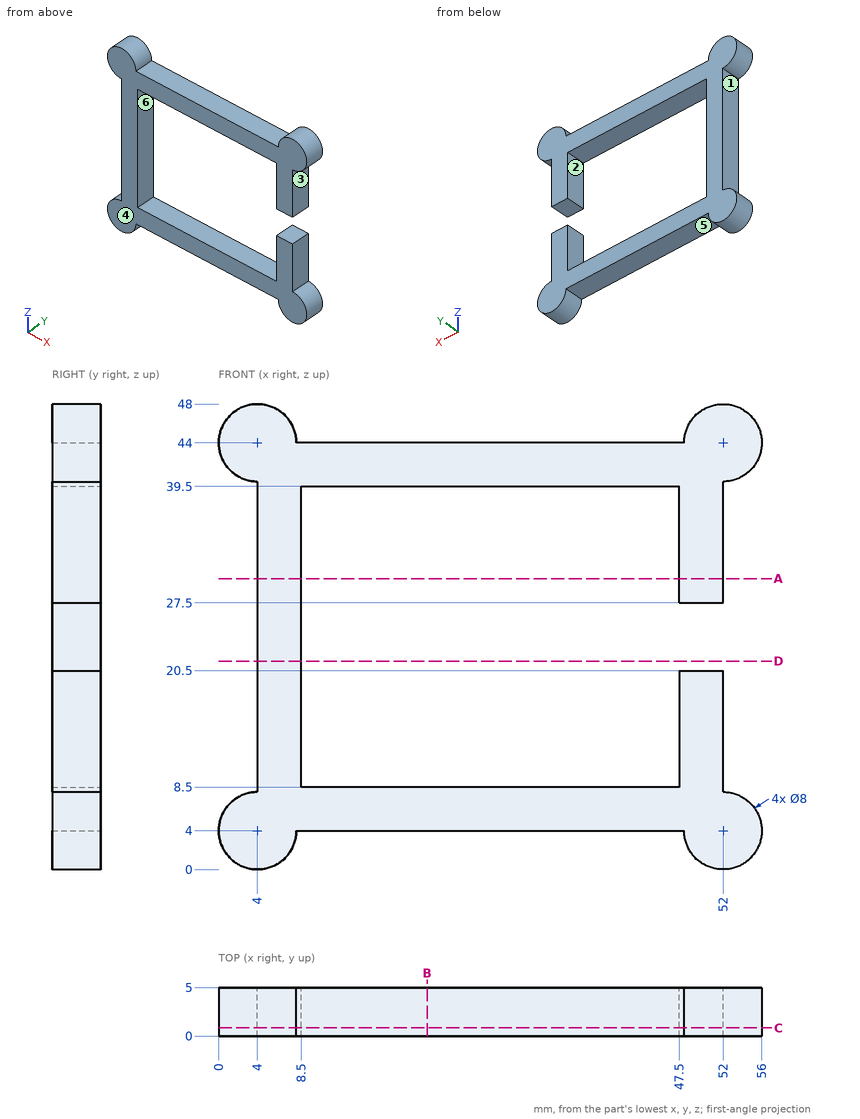
Could you check a few things on this drawing? It's one solid part, dimensions in mm from its lowest x, y, z. A direction names the side the tool comes from. Give positions to 0.01 mm unless a question says otherwise; leave off trailing zeros. Loops run counter-clockwise (first coordinate to the right, second up) from the corner with the lowest first, then second, coordinate; pieces in that order, holes last. Notation, with made-up numbers: (-2, 83) -> (20, 83) arc R23 cw to (20, 107) -> close; hole circle Ø5 at (-28, 24). An arc over 180 degrees is marked (long way). Use one line per item in the form item = value. Start each with the question number.
1) Imagine slicing it at C-C (y = 0.85). Please give me the cut outline in (x, z).
2) Imagine slicing it at A-A (z = 30). Please give me the cut outline in (x, y), then the cut area to 3 significant figures.
3) For P1, Ø1, axis at y = 0.5, z = 15.5, coming from the +X side; P2, Ø2.5, axis at y = 1.5, z = 14, coming from the -X side; P3, Ø10, axis at x = 34.5, z = 38.5, coming from the -Y side; P4, Ø1.3, axis at x = 50, y = 2, coming from the +Z side, each with a flat end and sliding along its axis, tell me the tip position at first contact or that it passes through.
4) Thinking about a two-plate mould opening in Z: for the marked faces 4, 5 and 6, which applies, +Z half, -Z half, draft (parallel to the pull), parting line (faces both ways), or undercut?
5) Imagine slicing it at D-D (z = 21.5). Please give me the cut outline in (x, y), then the cut area to 3 significant figures.
6) Which directions (+Z, -Z, +X, -X, +Y, -Y) give clear straight access to the entire face, cutting with the end or side of a thin tool? Please do the marked faces 1, 2 and 3.
7) Imagine slicing it at B-B (x = 21.5). Please give me the cut outline in (y, z).
8) Please list where these lines run through material, in increasing order: line 1 along X through (y, z) = (1.65, 36); line 2 along Z through (x, y) = (41.5, 0.65); line 3 along Z through (x, y) = (49, 2.8).
Check values:
q1.outline = (4, 8) arc R4 ccw (long way) to (8, 4) -> (48, 4) arc R4 ccw (long way) to (52, 8) -> (52, 20.5) -> (47.5, 20.5) -> (47.5, 8.5) -> (8.5, 8.5) -> (8.5, 39.5) -> (47.5, 39.5) -> (47.5, 27.5) -> (52, 27.5) -> (52, 40) arc R4 ccw (long way) to (48, 44) -> (8, 44) arc R4 ccw (long way) to (4, 40) -> close
q2.outline = (4, 0) -> (8.5, 0) -> (8.5, 5) -> (4, 5) -> close; (47.5, 0) -> (52, 0) -> (52, 5) -> (47.5, 5) -> close
q2.area = 45.0 mm^2
q3.P1 = 52
q3.P2 = 4
q3.P3 = 0
q3.P4 = 47.77
q4.face_4 = draft
q4.face_5 = -Z half
q4.face_6 = undercut
q5.outline = (4, 0) -> (8.5, 0) -> (8.5, 5) -> (4, 5) -> close
q5.area = 22.5 mm^2
q6.face_1 = -X, +Y, -Y
q6.face_2 = +Y, -Y
q6.face_3 = +X, +Y, -Y
q7.outline = (0, 4) -> (5, 4) -> (5, 8.5) -> (0, 8.5) -> close; (0, 39.5) -> (5, 39.5) -> (5, 44) -> (0, 44) -> close
q8.line_1 = 4 to 8.5, 47.5 to 52
q8.line_2 = 4 to 8.5, 39.5 to 44
q8.line_3 = 1.35 to 20.5, 27.5 to 46.65
